from build123d import *

# Parameters (mm, degrees)
PAD_DEPTH       = 5
CHAMFER_SIZE    = 1
CHAMFER001_SIZE = 1


with BuildPart() as part:
    # Sketch → Pad (new body)
    with BuildSketch(Plane.XY):
        with BuildLine():
            Line((57.783013, 41.350446), (57.783013, -41.350446))
            Line((-23.135408, -41.350446), (57.783013, -41.350446))
            Line((-23.135408, -21.854214), (-23.135408, -41.350446))
            Line((-40.557513, -38.160834), (-23.135408, -21.854214))
            Line((-55.820071, -21.854214), (-40.557513, -38.160834))
            Line((-55.820071, -41.438588), (-55.820071, -21.854214))
            Line((-55.820071, -41.438588), (-94.185086, -15.952922))
            ThreePointArc((-94.185086, 15.952922), (-102.739709, 0), (-94.185086, -15.952922))
            Line((-55.820071, 41.438588), (-94.185086, 15.952922))
            Line((-55.820071, 41.438588), (-55.820071, 22.499577))
            Line((-55.820071, 22.499577), (-40.584183, 38.541902))
            Line((-40.584183, 38.541902), (-23.692736, 22.499577))
            Line((-23.692736, 22.499577), (-23.692736, 41.350446))
            Line((-23.692736, 41.350446), (57.783013, 41.350446))
        make_face()
    extrude(amount=PAD_DEPTH)

    # Chamfer
    chamfer_edges = [part.edges().sort_by_distance(p)[0] for p in [
        (-55.820071, 31.969082, 5),
        (-48.202127, 30.52074, 5),
        (-32.138459, 30.52074, 5),
        (-23.692736, 31.925012, 5),
        (17.045139, 41.350446, 5),
        (57.783013, 0, 5),
        (17.323802, -41.350446, 5),
        (-23.135408, -31.60233, 5),
        (-31.846461, -30.007524, 5),
        (-48.188792, -30.007524, 5),
        (-55.820071, -31.646401, 5),
        (-75.002579, -28.695755, 5),
        (-102.739709, 0, 5),
        (-75.002579, 28.695755, 5),
    ]]
    chamfer(chamfer_edges, length=CHAMFER_SIZE)

    # Chamfer001
    chamfer001_edges = [part.edges().sort_by_distance(p)[0] for p in [
        (-55.820071, 31.969082, 0),
        (-75.002579, 28.695755, 0),
        (-48.202127, 30.52074, 0),
        (-32.138459, 30.52074, 0),
        (-23.692736, 31.925012, 0),
        (17.045139, 41.350446, 0),
        (57.783013, 0, 0),
        (17.323802, -41.350446, 0),
        (-31.846461, -30.007524, 0),
        (-48.188792, -30.007524, 0),
        (-55.820071, -31.646401, 0),
        (-75.002579, -28.695755, 0),
        (-102.739709, 0, 0),
    ]]
    chamfer(chamfer001_edges, length=CHAMFER001_SIZE)


solid = part.part
Can you work these out from the model? Positions are in its coordinate system, mm. A direction names the side the tool comes from. Round coordinates to 2 decimals unless told otherwise and drop trailing zeros. Order: outer loops, then holes, each group sorted by start corner. A loop starts at its lowest first (then second) coordinate and runs counter-clockwise, first axis right, second up. Notation, with made-up numbers: M 12,47.25 L 53,47.25 A24 cw 53,86.25 Z; hole C -29.75,82 d1. An arc over 180 degrees is marked long. Use a Markdown table: item, result.
1) Imagine slicing it at C-C (x = -69.5). List the corners of the cut face in (y, z) for me, then the cut area to 3 significant figures.
Geometry says:
| item | result |
|---|---|
| outline | M -32.35,1 L -31.15,0 L 31.15,0 L 32.35,1 L 32.35,4 L 31.15,5 L -31.15,5 L -32.35,4 Z |
| area | 321 mm² |
2) I'm going to push flat-ended pins straight in: P1, Ø2, axis at x = 40, z = 3.5, coming from the +Y side; P2, Ø1, axis at x = -51, z = 0.5, coming from the +Y side; P3, Ø2.5, axis at x = -2, z = 2.5, coming from the -Y side. Where does each tip first touch, or does it pass through?
Geometry says:
| item | result |
|---|---|
| P1 | stops at y = 41.35 |
| P2 | stops at y = 27.75 |
| P3 | stops at y = -41.35 |
3) If we mould it in two halves opening along X, with no side actions, what happens to faces 5 (the face through (-4, 1, 0)), 6 (the face through (-55.82, -32, 2)), 7 (the face through (57.783, 1, 2))? For each: +X half, -X half, draft (parallel to the pull), parting line (faces both ways), or undercut.
Geometry says:
| item | result |
|---|---|
| face 5 | draft |
| face 6 | undercut |
| face 7 | +X half |
4) Imagine slicing it at A-A (y = 25). List the corners of the cut face in (x, z) for me.
Geometry says:
| item | result |
|---|---|
| outline | M -80.57,1 L -78.76,0 L -56.82,0 L -55.82,1 L -55.82,4 L -56.82,5 L -78.76,5 L -80.57,4 Z; M -53.45,1 L -52.07,0 L -27.78,0 L -26.33,1 L -26.33,4 L -27.78,5 L -52.07,5 L -53.45,4 Z; M -23.69,1 L -22.69,0 L 56.78,0 L 57.78,1 L 57.78,4 L 56.78,5 L -22.69,5 L -23.69,4 Z |
5) If I drill on line 1 along X through (y, z) = (-33, 0.9); line 2 along X through (y, z) = (33, 1.5); line 3 along Y through (x, z) = (13.5, 1.35), over which ranges is the centre line in solid material (lowest first)?
Geometry says:
| item | result |
|---|---|
| line 1 | x = -68.34 to -55.92, -45.25 to -35.19, -23.14 to 57.68 |
| line 2 | x = -68.52 to -55.82, -45.85 to -34.75, -23.69 to 57.78 |
| line 3 | y = -41.35 to 41.35 |
6) Imagine slicing it at B-B (z = 1.95). List the corners of the cut face in (x, y) for me.
Geometry says:
| item | result |
|---|---|
| outline | M -94.19,-15.95 L -55.82,-41.44 L -55.82,-21.85 L -40.56,-38.16 L -23.14,-21.85 L -23.14,-41.35 L 57.78,-41.35 L 57.78,41.35 L -23.69,41.35 L -23.69,22.5 L -40.58,38.54 L -55.82,22.5 L -55.82,41.44 L -94.19,15.95 A19.15 ccw Z |
7) Imagine slicing it at D-D (y = -26). List the corners of the cut face in (x, z) for me.
Geometry says:
| item | result |
|---|---|
| outline | M -79.06,1 L -77.25,0 L -56.82,0 L -55.82,1 L -55.82,4 L -56.82,5 L -77.25,5 L -79.06,4 Z; M -51.94,1 L -50.57,0 L -29.03,0 L -27.56,1 L -27.56,4 L -29.03,5 L -50.57,5 L -51.94,4 Z; M -23.14,0 L 56.78,0 L 57.78,1 L 57.78,4 L 56.78,5 L -22.14,5 L -23.14,4 Z |
8) On a 3-axis mill with a long thin cutter (end or side, diameter ignored), from which of +Z, -Z, +X, -X, +Y, -Y can I reach the whole of each face in a straight line? I mean faces 1 (the face through (-32.257, 30.633, 2.479)), 2 (the face through (-31.5, -29, 4.5)), 3 (the face through (-48.83, 29.15, 0.51)), 4 (the face through (-31.97, -29.45, 0.51)). Say none if no direction works.
Geometry says:
| item | result |
|---|---|
| face 1 | +Z, -Z, +Y |
| face 2 | +Z, -Y |
| face 3 | -Z, +Y |
| face 4 | -Z, -Y |
